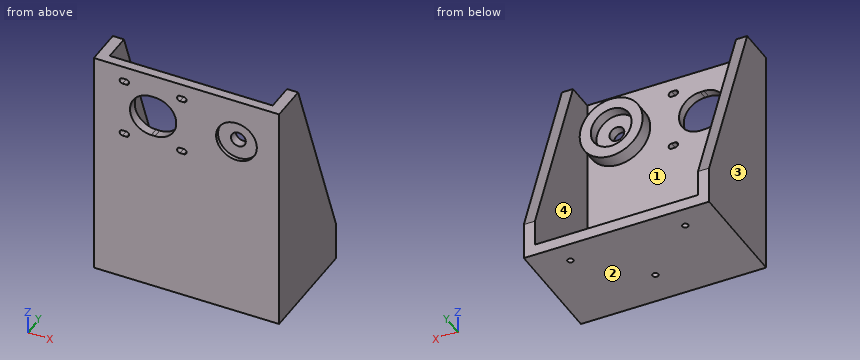
from build123d import *

# Parameters (mm, degrees)
CYLINDER040_R     = 11
CYLINDER040_DEPTH = 8
CYLINDER041_R     = 4
CYLINDER041_DEPTH = 34
CYLINDER046_R     = 1.6
CYLINDER046_DEPTH = 10
EXTRUDE031_DEPTH  = 10
CYLINDER039_R     = 11
CYLINDER039_DEPTH = 8
BOX010_W          = 88
BOX010_H          = 60
BOX010_DEPTH      = 128
EXTRUDE005_DEPTH  = 100
CYLINDER038_R     = 17
CYLINDER038_DEPTH = 8


with BuildPart() as cilindro040:
    # Cylinder040 → Cylinder040 (new body)
    with BuildSketch(Plane(origin=(203, 25, 2), x_dir=(1, 0, 0), z_dir=(0, 1, 0))):
        Circle(CYLINDER040_R)
    extrude(amount=CYLINDER040_DEPTH)


with BuildPart() as cilindro041:
    # Cylinder041 → Cylinder041 (new body)
    with BuildSketch(Plane(origin=(203, 8, 2), x_dir=(1, 0, 0), z_dir=(0, 1, 0))):
        Circle(CYLINDER041_R)
    extrude(amount=CYLINDER041_DEPTH)


with BuildPart() as cono:
    # Cone → Cone (revolve)
    with BuildSketch(Plane(origin=(0, 0, -96), x_dir=(1, 0, 0), z_dir=(0, -1, 0))):
        Polygon((0, 0), (1.6, 0), (4.1, 3), (0, 3), align=None)
    revolve(axis=Axis((0, 0, -96), (0, 0, 1)))


with BuildPart() as cilindro046:
    # Cylinder046 → Cylinder046 (new body)
    with BuildSketch(Plane.XY.offset(-106)):
        Circle(CYLINDER046_R)
    extrude(amount=CYLINDER046_DEPTH)


with BuildPart() as fusion030:
    # Fusion030 base: copy of Cilindro046
    add(cilindro046.part)

    # Fusion030: union Cono
    add(cono.part)


with BuildPart() as fusion030_1:
    # Fusion030 placement: moved
    add(fusion030.part.moved(Location((207, 66, 0))))


with BuildPart() as fusion031:
    # Fusion031 base: copy of Cilindro046
    add(cilindro046.part)

    # Fusion031: union Cono
    add(cono.part)


with BuildPart() as fusion031_1:
    # Fusion031 placement: moved
    add(fusion031.part.moved(Location((145, 66, 0))))


with BuildPart() as fusion032:
    # Fusion032 base: copy of Cilindro046
    add(cilindro046.part)

    # Fusion032: union Cono
    add(cono.part)


with BuildPart() as fusion032_1:
    # Fusion032 placement: moved
    add(fusion032.part.moved(Location((176, 37, 0))))


with BuildPart() as extrude031:
    # Sketch023 → Extrude031 (new body)
    with BuildSketch(Plane.XZ):
        with BuildLine():
            ThreePointArc((-1, 11.5), (-12.5, 0), (-1, -11.5))
            Line((-1, -11.5), (1, -11.5))
            ThreePointArc((1, -11.5), (12.5, 0), (1, 11.5))
            Line((-1, 11.5), (1, 11.5))
        make_face()
        with BuildLine():
            ThreePointArc((-16.5, 17.05), (-18.05, 15.5), (-16.5, 13.95))
            Line((-16.5, 13.95), (-14.5, 13.95))
            ThreePointArc((-14.5, 13.95), (-12.95, 15.5), (-14.5, 17.05))
            Line((-16.5, 17.05), (-14.5, 17.05))
        make_face()
        with BuildLine():
            ThreePointArc((14.5, 17.05), (12.95, 15.5), (14.5, 13.95))
            Line((14.5, 13.95), (16.5, 13.95))
            ThreePointArc((16.5, 13.95), (18.05, 15.5), (16.5, 17.05))
            Line((14.5, 17.05), (16.5, 17.05))
        make_face()
        with BuildLine():
            ThreePointArc((-16.5, -13.95), (-18.05, -15.5), (-16.5, -17.05))
            Line((-16.5, -17.05), (-14.5, -17.05))
            ThreePointArc((-14.5, -17.05), (-12.95, -15.5), (-14.5, -13.95))
            Line((-16.5, -13.95), (-14.5, -13.95))
        make_face()
        with BuildLine():
            ThreePointArc((14.5, -13.95), (12.95, -15.5), (14.5, -17.05))
            Line((14.5, -17.05), (16.499986, -17.05))
            ThreePointArc((16.499986, -17.05), (18.05, -15.500007), (16.5, -13.95))
            Line((14.5, -13.95), (16.5, -13.95))
        make_face()
    extrude(amount=EXTRUDE031_DEPTH)


with BuildPart() as extrude031_1:
    # Extrude031 placement: moved
    add(extrude031.part.moved(Location((158, 25, 2))))


with BuildPart() as fusion012:
    # Cylinder039 → Cylinder039 (new body)
    with BuildSketch(Plane(origin=(203, 12, 2), x_dir=(1, 0, 0), z_dir=(0, 1, 0))):
        Circle(CYLINDER039_R)
    extrude(amount=CYLINDER039_DEPTH)

    # Fusion012: union Cilindro040, Cilindro041, Fusion030, Fusion031, Fusion032, Extrude031
    add(cilindro040.part)
    add(cilindro041.part)
    add(fusion030_1.part)
    add(fusion031_1.part)
    add(fusion032_1.part)
    add(extrude031_1.part)


with BuildPart() as cubo009:
    # Box010 → Box010 (new body)
    with BuildSketch(Plane(origin=(132, 23, -93), x_dir=(1, 0, 0), z_dir=(0, 0, 1))):
        with Locations((44, 30)):
            Rectangle(BOX010_W, BOX010_H)
    extrude(amount=BOX010_DEPTH)


with BuildPart() as cut010:
    # Sketch005 → Extrude005 (new body)
    with BuildSketch(Plane.YZ.offset(126)):
        Polygon((18, 26), (18, -99), (78, -99), (78, -79), (38, 26), align=None)
    extrude(amount=EXTRUDE005_DEPTH)

    # Cut010: cut Cubo009
    add(cubo009.part, mode=Mode.SUBTRACT)


with BuildPart() as soporte_motor:
    # Cylinder038 → Cylinder038 (new body)
    with BuildSketch(Plane(origin=(203, 23, 2), x_dir=(1, 0, 0), z_dir=(0, 1, 0))):
        Circle(CYLINDER038_R)
    extrude(amount=CYLINDER038_DEPTH)

    # Fusion013: union Cut010
    add(cut010.part)

    # Cut008: cut Fusion012
    add(fusion012.part, mode=Mode.SUBTRACT)


with BuildPart() as soporte_motor_1:
    # Cut008 placement: moved
    add(soporte_motor.part.moved(Location((0, 13.5, 0))))


solid = soporte_motor_1.part
Source: CAD feature listing. Evaluate the final solid. Frame: model axes, mm. Face numbers are marked on the shaded views. Coordinates: 2 decimals unless noted, no trailing zeros. Loops run counter-clockwise (first coordinate to the right, second up) from the corner with the lowest first, then second, coordinate; pieces in that order, holes last. Notation, with made-up numbers: (-17, 14.25) -> (11, 14.25) arc R10 ccw to (11, 32.25) -> close; hole circle Ø8 at (-10, 26). An arc over 180 degrees is marked (long way). Answer in a Markdown table with one row per item. Add a question column.
Q1. Section C-C on x = 166.5. Return the cut outline in (y, z).
Q2. Contact query for flat-ended pins moving along their axis: pin 1 Ø11 at (x, z) = (202, 3) entering from -Y; pin 2 Ø4 at (x, z) = (153.5, -64) entering from +Y; pin 3 Ø2 at (x, y) = (142, 54.5) entering from +Z. Output: stop coordinate, or through.
Q3. Section D-D on z = -43. Return the cut outline in (x, y).
Q4. Pull-direction query (Z, two-part tool) for the marked faces 1, 2, 3 and 4; classes: pulls with the +Z half, pulls with the -Z half, needs draft (parallel to the pull), parting line crosses it, or undercut.
Q5. Ray query, line 1 along Z through (x, y) = (203, 41); line 2 along Z through (x, y) = (203, 36.6); line 3 along Y through (x, z) = (176, -97.9). Return the intervals inside material, ascending.
Q6. Section A-A on y = 79.5. Return the cut outline in (x, z).
Computed values:
| question | item | result |
|---|---|---|
| 1 | outline | (31.5, -99) -> (91.5, -99) -> (91.5, -93) -> (36.5, -93) -> (36.5, -6.72) -> (31.5, -6.72) -> close; (31.5, 10.72) -> (36.5, 10.72) -> (36.5, 26) -> (31.5, 26) -> close |
| 2 | pin 1 | stops at y = 33.5 |
| 2 | pin 2 | stops at y = 36.5 |
| 2 | pin 3 | stops at z = -93 |
| 3 | outline | (126, 31.5) -> (226, 31.5) -> (226, 77.79) -> (220, 77.79) -> (220, 36.5) -> (132, 36.5) -> (132, 77.79) -> (126, 77.79) -> close |
| 4 | face 1 | undercut |
| 4 | face 2 | pulls with the -Z half |
| 4 | face 3 | needs draft |
| 4 | face 4 | undercut |
| 5 | line 1 | z = -99 to -93, -15 to -9, 13 to 19 |
| 5 | line 2 | z = -99 to -93, -15 to -2, 6 to 19 |
| 5 | line 3 | y = 31.5 to 48.9, 52.1 to 91.5 |
| 6 | outline | (126, -99) -> (143.4, -99) -> (143.4, -96) -> (140.9, -93) -> (132, -93) -> (132, -47.5) -> (126, -47.5) -> close; (146.6, -99) -> (205.4, -99) -> (205.4, -96) -> (202.9, -93) -> (149.1, -93) -> (146.6, -96) -> close; (208.6, -99) -> (226, -99) -> (226, -47.5) -> (220, -47.5) -> (220, -93) -> (211.1, -93) -> (208.6, -96) -> close |
